Autodesk Fusion 360 part; units mm, degrees
sketch "ESP32 Devkit Board" plane through (0, 0, 0) normal (0, 0, 1) x (1, 0, 0)
  line L0 (0, 0) -> (-66, 0)
  line L1 (-66, 0) -> (-66, 63)
  line L2 (-66, 63) -> (0, 63)
  line L3 (0, 63) -> (0, 0)
  circle A0 centre (-63, 60) radius 1.5
  circle A1 centre (-3, 60) radius 1.5
  circle A2 centre (-3, 3) radius 1.5
  circle A3 centre (-63, 3) radius 1.5
  line L4 (-67.9, 17) -> (-89, 17)
  line L5 (-89, 17) -> (-89, 60)
  line L6 (-89, 60) -> (-67.9, 60)
  line L7 (-67.9, 60) -> (-67.9, 17)
  circle A4 centre (-70.4, 54) radius 1.5
  circle A5 centre (-86.5, 23) radius 1.5
  line L8 (13, 0) -> (67, 0)
  line L9 (67, 0) -> (67, 82.5)
  line L10 (67, 82.5) -> (13, 82.5)
  line L11 (13, 82.5) -> (13, 0)
  line L12 (-100, -5) -> (72, -5)
  line L13 (72, -5) -> (72, 88)
  line L14 (72, 88) -> (-100, 88)
  line L15 (-100, 88) -> (-100, -5)
  line L16 (12, -1) -> (22, -1)
  line L17 (22, -1) -> (22, 9)
  line L18 (22, 9) -> (12, 9)
  line L19 (12, 9) -> (12, -1)
  line L20 (68, -1) -> (58, -1)
  line L21 (58, -1) -> (58, 9)
  line L22 (58, 9) -> (68, 9)
  line L23 (68, 9) -> (68, -1)
  line L24 (69, 85) -> (59, 85)
  line L25 (59, 85) -> (59, 75)
  line L26 (59, 75) -> (69, 75)
  line L27 (69, 75) -> (69, 85)
  line L28 (11, 85) -> (21, 85)
  line L29 (21, 85) -> (21, 75)
  line L30 (21, 75) -> (11, 75)
  line L31 (11, 75) -> (11, 85)
  line L32 (-103, 91) -> (75, 91)
  line L33 (75, 91) -> (75, -8)
  line L34 (75, -8) -> (-103, -8)
  line L35 (-103, -8) -> (-103, 91)
  dimension "d1" = 66
  dimension "d2" = 63
  dimension "d3" = 3
  dimension "d4" = 3
  dimension "d5" = 3
  dimension "d6" = 3
  dimension "d7" = 3
  dimension "d8" = 3
  dimension "d9" = 3
  dimension "d10" = 3
  dimension "d11" = 3
  dimension "d12" = 3
  dimension "d13" = 3
  dimension "d14" = 3
  dimension "d15" = 21.1
  dimension "d16" = 43
  dimension "d17" = 3
  dimension "d18" = 6
  dimension "d19" = 2.5
  dimension "d20" = 3
  dimension "d21" = 2.5
  dimension "d22" = 6
  dimension "d23" = 54
  dimension "d24" = 82.5
  dimension "d69" = 10
  dimension "d70" = 10
  dimension "d71" = 10
  dimension "d72" = 10
  dimension "d73" = 10
  dimension "d74" = 10
  dimension "d75" = 10
  dimension "d76" = 10
extrude "Extrude1" add sketch "ESP32 Devkit Board" along normal blind 1 contours L0 L1 L2 L3 | A0 | A1 | A2 | A3 | L4 L5 L6 L7 | A4 | A5 | L8 L11 L17 L18 | L8 L11 L16 L17 L18 L19 | L8 L9 L10 L11 L17 L18 L21 L22 L25 L26 L29 L30 | L8 L9 L21 L22 | L8 L9 L20 L21 L22 L23 | L10 L11 L28 L29 L30 L31 | L10 L11 L29 L30 | L9 L10 L25 L26 | L9 L10 L24 L25 L26 L27 | L12 L13 L14 L15 makes body 1
extrude "Extrude2" add sketch "ESP32 Devkit Board" along normal blind 6 separate body contours A4 makes body 2
extrude "Extrude3" add sketch "ESP32 Devkit Board" along normal blind 6 separate body contours A5 makes body 3
extrude "Extrude4" add sketch "ESP32 Devkit Board" along normal blind 6 separate body contours A0 | A1 | A2 | A3 makes body 4 at (-4.3173, 60.7174, 4) makes body 5 at (-1.5019, 2.9252, 4) makes body 6 at (-61.7201, 60.7822, 4) makes body 7 at (-62.5937, 4.4439, 4)
move_face "OffsetFaces1" offset 1 1 faces at (-85.5075, 24.1247, 4) on bodies 3
move_face "OffsetFaces2" offset 1 1 faces at (-62.5937, 4.4439, 4) on bodies 7
move_face "OffsetFaces3" offset 1 1 faces at (-69.4075, 55.1247, 4) on bodies 2
move_face "OffsetFaces4" offset 1 1 faces at (-61.7201, 60.7822, 4) on bodies 6
move_face "OffsetFaces5" offset 1 1 faces at (-4.3173, 60.7174, 4) on bodies 4
move_face "OffsetFaces6" offset 1 1 faces at (-1.5019, 2.9252, 4) on bodies 5
hole "Hole1" at (-63, 60, 0) direction (0, 0, 1) diameter 2.529 depth 16 tip angle 118 bodies 1 6
hole "Hole2" at (-3, 60, 0) direction (0, 0, 1) diameter 2.529 depth 16 tip angle 118 bodies 1 4
hole "Hole3" at (-86.5, 23, 0) direction (0, 0, 1) diameter 2.529 depth 29 tip angle 118 bodies 1 3
hole "Hole4" at (-70.4, 54, 0) direction (0, 0, 1) diameter 2.529 depth 29 tip angle 118 bodies 1 2
hole "Hole5" at (-3, 3, 0) direction (0, 0, 1) diameter 2.529 depth 29 tip angle 118 bodies 1 5
hole "Hole6" at (-63, 3, 0) direction (0, 0, 1) diameter 2.529 depth 29 tip angle 118 bodies 1 7
extrude "Extrude5" add sketch "ESP32 Devkit Board" along normal blind 10 separate body contours L8 L11 L16 L17 L18 L19 | L8 L9 L20 L21 L22 L23 | L10 L11 L28 L29 L30 L31 | L9 L10 L24 L25 L26 L27 makes body 8 at (65.6667, 85, 3.3333) makes body 9 at (15.3333, -1, 3.3333) makes body 10 at (68, 5.6667, 3.3333) makes body 11 at (11, 78.3333, 3.3333)
extrude "Extrude6" add sketch "ESP32 Devkit Board" along normal blind 30 contours L32 L33 L34 L35 bodies 1
sketch "Sketch2" plane through (0, -8, 0) normal (0, -1, 0) x (1, 0, 0)
  line L0 (-103, 0) -> (75, 0)
  line L1 (75, 0) -> (75, 30)
  line L2 (75, 30) -> (-103, 30)
  line L3 (-103, 30) -> (-103, 0)
  circle A0 centre (60, 15) radius 1.4142
  circle A1 centre (50, 15) radius 1
  circle A2 centre (40, 15) radius 1.4923
  circle A3 centre (30, 15) radius 1.4142
  line L4 (-91, 15) -> (-80, 15)
  line L5 (-80, 15) -> (-80, 9)
  line L6 (-80, 9) -> (-91, 9)
  line L7 (-91, 9) -> (-91, 15)
  dimension "d81" = 11
  dimension "d82" = 6
hole "Hole7" at (30, -8, 15) at (40, -8, 15) at (50, -8, 15) at (60, -8, 15) direction (0, 1, 0) diameter 3.8 depth 3 tip angle 118 bodies 1
extrude "Extrude7" cut sketch "Sketch2" against normal blind 9 contours L4 L5 L6 L7 bodies 1
extrude "Extrude8" add sketch "ESP32 Devkit Board" against normal blind 5 contours L0 L1 L2 L3 | A0 | A1 | A2 | A3 | L4 L5 L6 L7 | A4 | A5 | L8 L11 L17 L18 | L8 L11 L16 L17 L18 L19 | L8 L9 L10 L11 L17 L18 L21 L22 L25 L26 L29 L30 | L8 L9 L21 L22 | L8 L9 L20 L21 L22 L23 | L10 L11 L28 L29 L30 L31 | L10 L11 L29 L30 | L9 L10 L25 L26 | L9 L10 L24 L25 L26 L27 | L12 L13 L14 L15 | L32 L33 L34 L35 bodies 1 2 3 4 5 6 7 8 9 10 11
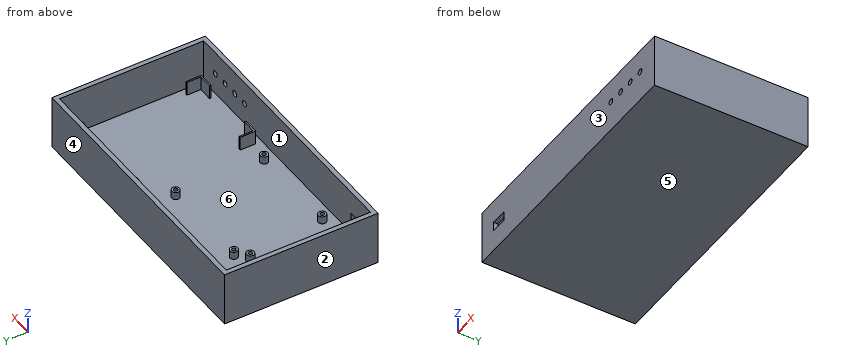
Build history of the part. All positions in model axes, mm. Face numbers are marked on the shaded views. A direction names the side the tool comes from. Round coordinates to 2 decimals unless told otherwise and drop trailing zeros. Write each loop counter-clockwise with the first axis right and the second up, starting at its lowest first coordinate (ties: lowest second). Pieces come first, ordered by that corner, then holes.
1) Band-saw the part on A-A, the plane z = 20.5. List the corners of the cut face in (x, y).
2) Mould opens along Y. For the marked faces 3, 4, 5 and 6 say: +Y half, -Y half, draft (parallel to the pull), parting line (faces both ways), or undercut.
3) Band-saw the part on B-B, the plane x = 50. List the corners of the cut face in (y, z), and give its area (3 significant figures).
4) 3-axis set-ups, long thin cutter, end or side, ignore diameter. For the marked faces 1 and 2: which of +Z, -Z, +X, -X, +Y, -Y reach the whole face in a straight line?
5) Drill centre lines: probe 1 along X at (y, z) = (23, 2); probe 2 along Y at (x, z) = (-63, 1.3); probe 3 along X at (y, z) = (60, 2.15). Where is each one in solid material? Low to high.
6) Pin check, flat tips, straight feed: pin 1 (3 mm diameter, centred on x = -86.5, y = 22.5, fed in from +Z); pin 2 (6 mm diameter, centred on x = 17, y = 53.5, fed in from +Z). Stop position of each tip, or through.
7) Band-saw the part on C-C, the plane y = 72.5. List the corners of the cut face in (x, z), and give its area (3 significant figures).
8) Band-saw the part on D-D, the plane z = 4. Give the number of separate pieces and of enclosed holes in the cut face, and give its area (3 significant figures).
Ans:
1. outline: (-103, -8) - (75, -8) - (75, 91) - (-103, 91) - close; hole (-100, -5) - (72, -5) - (72, 88) - (-100, 88) - close
2. face 3: -Y half
2. face 4: +Y half
2. face 5: draft
2. face 6: undercut
3. outline: (-8, -5) - (91, -5) - (91, 30) - (88, 30) - (88, 1) - (-5, 1) - (-5, 13.1) - (-8, 13.1) - close; (-8, 16.9) - (-5, 16.9) - (-5, 30) - (-8, 30) - close
3. area: 757 mm2
4. face 1: +Z
4. face 2: +Z, -Z, -X, +Y, -Y
5. probe 1: x = -103 to -100, -89 to -87.76, -85.24 to -84, 72 to 75
5. probe 2: y = -8 to -5, 0.5 to 1.74, 4.26 to 5.5, 57.5 to 58.74, 61.26 to 62.5, 88 to 91
5. probe 3: x = -103 to -100, -65.5 to -64.26, -61.74 to -60.5, -5.5 to -4.26, -1.74 to -0.5, 72 to 75
6. pin 1: stops at z = 6
6. pin 2: stops at z = 1
7. outline: (-103, -5) - (75, -5) - (75, 30) - (72, 30) - (72, 1) - (-100, 1) - (-100, 30) - (-103, 30) - close
7. area: 1,240 mm2
8. separate pieces: 11
8. enclosed holes: 7
8. area: 1,830 mm2
